Work out the finished part from the listing and answer in its coordinate system (mm). Face numbers are marked on the shaded views. A direction names the side the tool comes from. Coordinates: 2 decimals unless noted, no trailing zeros. Loops run counter-clockwise (first coordinate to the right, second up) from the corner with the lowest first, then second, coordinate; pieces in that order, holes last. Notation, with made-up numbers: (-25.75, 70) -> (-10.75, 70) arc R3 cw to (-10.75, 75) -> close; hole circle Ø6 at (10.5, 67.25). An arc over 180 degrees is marked (long way). Use a Markdown table: item, result.
from build123d import *

# Parameters (mm, degrees)
CYLINDER058_R               = 3
CYLINDER058_DEPTH           = 14
CYLINDER059_R               = 4
CYLINDER059_DEPTH           = 14
CYLINDER057_R               = 3
CYLINDER057_DEPTH           = 25
CYLINDER057_ROLL_ANGLE      = -80.307838
CYLINDER057_PITCH_ANGLE     = -6.032922
CYLINDER057_PLACEMENT_ANGLE = 60.76787
CYLINDER055_R               = 4
CYLINDER055_DEPTH           = 23
CYLINDER055_ROLL_ANGLE      = -80.242002
CYLINDER055_PITCH_ANGLE     = -5.711725
CYLINDER055_PLACEMENT_ANGLE = 60.604575
CYLINDER056_R               = 3
CYLINDER056_DEPTH           = 20
CYLINDER056_ROLL_ANGLE      = -80.307852
CYLINDER056_PITCH_ANGLE     = -6.032925
CYLINDER056_PLACEMENT_ANGLE = 60.767852
BOX022_W                    = 25
BOX022_H                    = 8
BOX022_DEPTH                = 20
BOX022_PLACEMENT_ANGLE      = 47
BOX021_W                    = 4
BOX021_H                    = 17
BOX021_DEPTH                = 20
BOX021_PLACEMENT_ANGLE      = 47


with BuildPart() as cylindre054:
    # Cylinder058 → Cylinder058 (new body)
    with BuildSketch(Plane(origin=(-18, 17, -67), x_dir=(1, 0, 0), z_dir=(0, 0, 1))):
        Circle(CYLINDER058_R)
    extrude(amount=CYLINDER058_DEPTH)


with BuildPart() as cylindre055:
    # Cylinder059 → Cylinder059 (new body)
    with BuildSketch(Plane(origin=(-18, 17, -67), x_dir=(1, 0, 0), z_dir=(0, 0, 1))):
        Circle(CYLINDER059_R)
    extrude(amount=CYLINDER059_DEPTH)


with BuildPart() as cylindre053:
    # Cylinder057 → Cylinder057 (new body)
    with BuildSketch(Plane.XY):
        Circle(CYLINDER057_R)
    extrude(amount=CYLINDER057_DEPTH)


with BuildPart() as cylindre053_1:
    # Cylinder057 roll: moved
    add(cylindre053.part.rotate(Axis((0, 0, 0), (1, 0, 0)), CYLINDER057_ROLL_ANGLE))


with BuildPart() as cylindre053_2:
    # Cylinder057 pitch: moved
    add(cylindre053_1.part.rotate(Axis((0, 0, 0), (0, 1, 0)), CYLINDER057_PITCH_ANGLE))


with BuildPart() as cylindre053_3:
    # Cylinder057 placement: moved
    add(cylindre053_2.part.moved(Location((-3, 6, -72))).rotate(Axis((-3, 6, -72), (0, 0, 1)), CYLINDER057_PLACEMENT_ANGLE))


with BuildPart() as cut039:
    # Cylinder055 → Cylinder055 (new body)
    with BuildSketch(Plane.XY):
        Circle(CYLINDER055_R)
    extrude(amount=CYLINDER055_DEPTH)


with BuildPart() as cut039_1:
    # Cylinder055 roll: moved
    add(cut039.part.rotate(Axis((0, 0, 0), (1, 0, 0)), CYLINDER055_ROLL_ANGLE))


with BuildPart() as cut039_2:
    # Cylinder055 pitch: moved
    add(cut039_1.part.rotate(Axis((0, 0, 0), (0, 1, 0)), CYLINDER055_PITCH_ANGLE))


with BuildPart() as cut039_3:
    # Cylinder055 placement: moved
    add(cut039_2.part.moved(Location((-3, 6, -72))).rotate(Axis((-3, 6, -72), (0, 0, 1)), CYLINDER055_PLACEMENT_ANGLE))

    # Cut038: cut Cylindre053
    add(cylindre053_3.part, mode=Mode.SUBTRACT)


with BuildPart() as cut039_4:
    # Cut038 placement: moved
    add(cut039_3.part.moved(Location((2, 2, 1))))

    # Fusion027: union Cylindre055
    add(cylindre055.part)

    # Cut039: cut Cylindre054
    add(cylindre054.part, mode=Mode.SUBTRACT)


with BuildPart() as cylindre052:
    # Cylinder056 → Cylinder056 (new body)
    with BuildSketch(Plane.XY):
        Circle(CYLINDER056_R)
    extrude(amount=CYLINDER056_DEPTH)


with BuildPart() as cylindre052_1:
    # Cylinder056 roll: moved
    add(cylindre052.part.rotate(Axis((0, 0, 0), (1, 0, 0)), CYLINDER056_ROLL_ANGLE))


with BuildPart() as cylindre052_2:
    # Cylinder056 pitch: moved
    add(cylindre052_1.part.rotate(Axis((0, 0, 0), (0, 1, 0)), CYLINDER056_PITCH_ANGLE))


with BuildPart() as cylindre052_3:
    # Cylinder056 placement: moved
    add(cylindre052_2.part.moved(Location((3, 6, -72))).rotate(Axis((3, 6, -72), (0, 0, 1)), CYLINDER056_PLACEMENT_ANGLE))


with BuildPart() as cube022:
    # Box022 → Box022 (new body)
    with BuildSketch(Plane.XY):
        with Locations((12.5, 4)):
            Rectangle(BOX022_W, BOX022_H)
    extrude(amount=BOX022_DEPTH)


with BuildPart() as cube022_1:
    # Box022 placement: moved
    add(cube022.part.moved(Location((-10, -5, -81))).rotate(Axis((-10, -5, -81), (0, 0, 1)), BOX022_PLACEMENT_ANGLE))


with BuildPart() as fusion028:
    # Box021 → Box021 (new body)
    with BuildSketch(Plane.XY):
        with Locations((2, 8.5)):
            Rectangle(BOX021_W, BOX021_H)
    extrude(amount=BOX021_DEPTH)


with BuildPart() as fusion028_1:
    # Box021 placement: moved
    add(fusion028.part.moved(Location((-11, -9, -81))).rotate(Axis((-11, -9, -81), (0, 0, 1)), BOX021_PLACEMENT_ANGLE))

    # Fusion023: union Cube022
    add(cube022_1.part)

    # Cut037: cut Cylindre052
    add(cylindre052_3.part, mode=Mode.SUBTRACT)

    # Fusion028: union Cut039
    add(cut039_4.part)


solid = fusion028_1.part
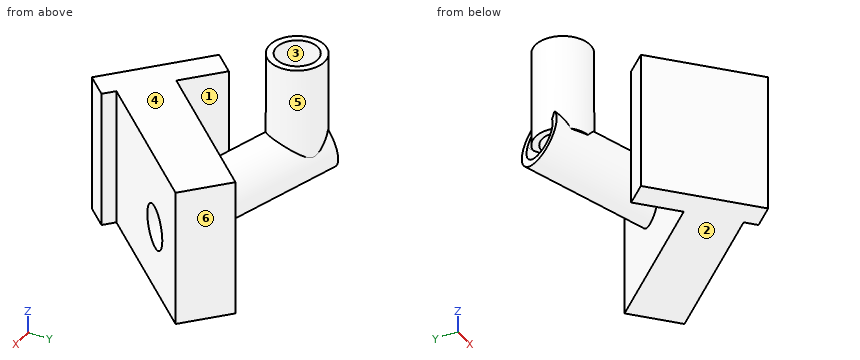
Q1. Determine the mould class of the marked faces 4, 5 and 6 for opening direction Y: pulls with the +Y half, pulls with the -Y half, needs draft (parallel to the pull), parting line crosses it, or undercut.
Solved:
| item | result |
|---|---|
| face 4 | needs draft |
| face 5 | undercut |
| face 6 | pulls with the +Y half |
Q2. For the marked faces 1, 2 and 3, determine the directions among +Z, -Z, +X, -X, +Y, -Y from which every point of the face is accessible in a straight line to the end or side of a thin tool.
Solved:
| item | result |
|---|---|
| face 1 | +Z, -Z |
| face 2 | -Z, +X, -X, +Y, -Y |
| face 3 | +Z |
Q3. Section B-B on z = -56 is taken. Determine the outline of the cut face in (x, y).
Solved:
| item | result |
|---|---|
| outline | circle Ø8 at (-18, 17); hole circle Ø6 at (-18, 17) |
Q4. Consider line 1 (X direction, y = 17, z = -58.5); line 2 (Y direction, x = -18, z = -62.75); line 3 (Y direction, x = -18, z = -58.75). Determine where each line is inside the solid, lowest interval first. Write a range as [from, to].
Solved:
| item | result |
|---|---|
| line 1 | [-22, -21], [-15, -14] |
| line 2 | [-2.47, 3], [13, 14], [20, 21] |
| line 3 | [13, 14], [20, 21] |
Q5. Section A-A on y = 17 is taken. State how many separate pieces and enclosed holes the cut face has, and give its area (3 significant figures).
Solved:
| item | result |
|---|---|
| separate pieces | 3 |
| enclosed holes | 0 |
| area | 123 mm² |
Q6. Given pin 1 Ø1.4 at (x, y) = (-19.5, 14) entering from -Z; pin 2 Ø10 at (x, z) = (-13.5, -64) entering from +Y; pin 3 Ø12 at (x, y) = (-11, -2) entering from +Z, each flat-ended and moving along its own axis, determine where each tip first touches the part or whether it passes through.
Solved:
| item | result |
|---|---|
| pin 1 | z = -70.61 |
| pin 2 | y = 21.56 |
| pin 3 | z = -61 |
